For this review, use the dimensioned drawing (mm, ordinates from the lowest corner) and the shaded views. Give positions to 0.01 mm unless a question says otherwise; leave off trailing zeros. Loops run counter-clockwise (first coordinate to the right, second up) from the corner with the lowest first, then second, coordinate; pieces in that order, holes last. Notation, with made-up numbers: (-4.5, -19.5) -> (33.5, -19.5) arc R23 ccw to (33.5, 19.5) -> close; hole circle Ø2 at (7.5, 70). An arc over 180 degrees is marked (long way). Write each question's results on one line, items separated by ' | '. Start each with the question number.
Q1. Wall thickness on L1, parallel to X at y = 26, z = 41.5; L2, parallel to X at y = 13, z = 83: over which ranges is each line inside the solid? List them lowest first. Write a range as [from, to].
Q2. Insertion check: pin 1 Ø4 at (y, z) = (106.5, 28.5) entering from +X; pin 2 Ø6 at (x, y) = (37, 23) entering from -Z; pin 3 Ø2 at (y, z) = (69, 34.5) entering from -X; pin 4 Ø1 at (y, z) = (15.5, 85) entering from +X. Each pin has a flat end and moves straight along its axis. Give the tip position at first contact, or say it passes through.
Q3. We need section A-A (y = 48). Write out the cut boundary in (x, z).
Q4. We need section B-B (z = 59). Write out the cut boundary in (x, y), plus the area to 3 significant figures.
Q5. We need section C-C (x = 15). Write out the cut boundary in (y, z), plus the area to 3 significant figures.
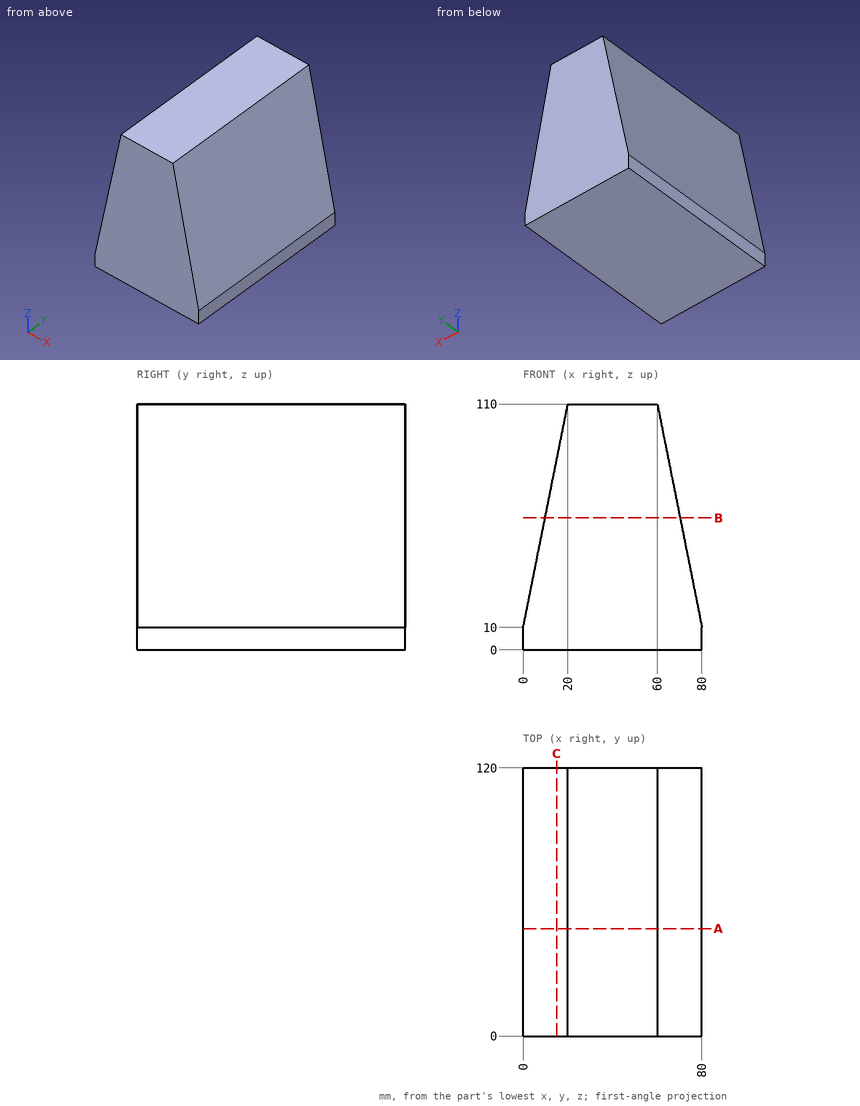
Output:
1) L1: [6.3, 73.7] | L2: [14.6, 65.4]
2) pin 1: x = 76.7 | pin 2: z = 0 | pin 3: x = 4.7 | pin 4: x = 65.1
3) outline: (0, 0) -> (80, 0) -> (80, 10) -> (60, 110) -> (20, 110) -> (0, 10) -> close
4) outline: (9.8, 0) -> (70.2, 0) -> (70.2, 120) -> (9.8, 120) -> close | area: 7,250 mm2
5) outline: (0, 0) -> (120, 0) -> (120, 85) -> (0, 85) -> close | area: 10,200 mm2
